Could you check a few things on this model? Use its own coordinates, in mm. A direction names the side the tool comes from. Give positions to 0.01 mm unless a question says otherwise; leave off trailing zeros. Write each loop counter-clockwise with the first axis right and the second up, starting at its lowest first coordinate (ties: lowest second). Pieces come first, ordered by that corner, then holes. Notation, with made-up numbers: (-17.5, 53.5) - (2.5, 53.5) arc R14 cw to (2.5, 78.5) - close; hole circle Ø5 at (86.25, -39). An arc over 180 degrees is marked (long way). Use one line per item in the form item = value.
```python
from build123d import *

# Parameters (mm, degrees)
SKETCH1_W           = 17.145
SKETCH1_H           = 17.145
BOSS_EXTRUDE1_DEPTH = 5.08
SKETCH2_R           = 1.27
CUT_EXTRUDE1_DEPTH  = 25.773139688
SKETCH3_R           = 2.54
CUT_EXTRUDE4_DEPTH  = 2.54
SKETCH4_W           = 6.307704678
SKETCH4_H           = 17.145
BOSS_EXTRUDE2_DEPTH = 17.78
SKETCH5_W           = 2.54
SKETCH5_H           = 17.145
BOSS_EXTRUDE3_DEPTH = 5.08
CHAMFER1_SIZE       = 3.175
BOSS_EXTRUDE4_DEPTH = 2.54
BOSS_EXTRUDE5_DEPTH = 2.54
SKETCH9_W           = 1
SKETCH9_H           = 17.145
CUT_EXTRUDE5_DEPTH  = 17.78
EXTRUDE_1_DEPTH     = 1
EXTRUDE_2_DEPTH     = 1
EXTRUDE_3_DEPTH     = 5.31
CUT_EXTRUDE_1_DEPTH = 44.874772364
CUT_EXTRUDE_2_DEPTH = 44.874772364
EXTRUDE_4_DEPTH     = 2.655
EXTRUDE_5_DEPTH     = 6.915
EXTRUDE_6_DEPTH     = 6.92


with BuildPart() as part:
    # Sketch1 → Boss-Extrude1 (new body)
    with BuildSketch(Plane.XY):
        with Locations((8.5725, -8.5725)):
            Rectangle(SKETCH1_W, SKETCH1_H)
    extrude(amount=BOSS_EXTRUDE1_DEPTH)

    # Sketch2 → Cut-Extrude1 (cut, through all)
    with BuildSketch(Plane(origin=(0, 0, 0), x_dir=(-1, 0, 0), z_dir=(0, 0, -1))):
        with Locations((-8.89, -2.5908)):
            Circle(SKETCH2_R)
        with Locations((-8.89, -14.5288)):
            Circle(SKETCH2_R)
    extrude(amount=-CUT_EXTRUDE1_DEPTH, mode=Mode.SUBTRACT)

    # Sketch3 → Cut-Extrude4 (cut)
    with BuildSketch(Plane(origin=(0, 0, 0), x_dir=(-1, 0, 0), z_dir=(0, 0, -1))):
        with Locations((-8.89, -2.5908)):
            Circle(SKETCH3_R)
        with Locations((-8.89, -14.5288)):
            Circle(SKETCH3_R)
    extrude(amount=-CUT_EXTRUDE4_DEPTH, mode=Mode.SUBTRACT)

    # Sketch4 → Boss-Extrude2 (add)
    with BuildSketch(Plane(origin=(0, 0, 0), x_dir=(-1, 0, 0), z_dir=(0, 0, -1))):
        with Locations((-3.153852339, -8.5725)):
            Rectangle(SKETCH4_W, SKETCH4_H)
    extrude(amount=BOSS_EXTRUDE2_DEPTH)

    # Sketch5 → Boss-Extrude3 (add)
    with BuildSketch(Plane.ZY):
        with Locations((3.81, -8.5725)):
            Rectangle(SKETCH5_W, SKETCH5_H)
    extrude(amount=BOSS_EXTRUDE3_DEPTH)

    # Chamfer1
    chamfer1_edges = [part.edges().sort_by_distance(p)[0] for p in [
        (0, -8.5725, -17.78),
    ]]
    chamfer(chamfer1_edges, length=CHAMFER1_SIZE)

    # Sketch7 → Boss-Extrude4 (add)
    with BuildSketch(Plane(origin=(0, 0, 0), x_dir=(1, 0, 0), z_dir=(0, 1, 0))):
        Polygon((-5.08, -2.54), (0, 14.605), (0, -2.54), align=None)
    extrude(amount=-BOSS_EXTRUDE4_DEPTH)

    # Sketch8 → Boss-Extrude5 (add)
    with BuildSketch(Plane.XZ.offset(17.145)):
        Polygon((0, 2.54), (-5.08, 2.54), (0, -14.605), align=None)
    extrude(amount=-BOSS_EXTRUDE5_DEPTH)

    # Sketch9 → Cut-Extrude5 (cut)
    with BuildSketch(Plane(origin=(0, 0, -17.78), x_dir=(-1, 0, 0), z_dir=(0, 0, -1))):
        with Locations((-5.807704678, -8.5725)):
            Rectangle(SKETCH9_W, SKETCH9_H)
    extrude(amount=-CUT_EXTRUDE5_DEPTH, mode=Mode.SUBTRACT)

    # 草图1 → 凸台-拉伸1 (add)
    with BuildSketch(Plane(origin=(0, 0, 0), x_dir=(1, 0, 0), z_dir=(0, 1, 0))):
        Polygon((17.145, 0), (5.307704678, 0), (5.307704678, 17.78), (3.175, 17.78), (0, 14.605), (-5.08, -2.54), (-5.08, -5.08), (17.145, -5.08), align=None)
    extrude(amount=EXTRUDE_1_DEPTH)

    # 草图2 → 凸台-拉伸2 (add)
    with BuildSketch(Plane.XZ.offset(17.145)):
        Polygon((5.307704678, -17.78), (5.307704678, 0), (17.145, 0), (17.145, 5.08), (-5.08, 5.08), (-5.08, 2.54), (0, -14.605), (3.175, -17.78), align=None)
    extrude(amount=EXTRUDE_2_DEPTH)

    # 草图3 → 凸台-拉伸3 (add)
    with BuildSketch(Plane(origin=(17.145, 0, 0), x_dir=(0, 0, -1), z_dir=(1, 0, 0))):
        Polygon((17.78, -18.145), (35.56, -18.145), (35.56, 1), (17.78, 1), (0, 1), (0, -18.145), align=None)
    extrude(amount=-EXTRUDE_3_DEPTH)

    # 草图4 → 切除-拉伸1 (cut, through all)
    with BuildSketch(Plane(origin=(0, 1, 0), x_dir=(1, 0, 0), z_dir=(0, 1, 0))):
        Polygon((15.015, 35.56), (11.835, 32.38), (11.835, 35.56), align=None)
    extrude(amount=-CUT_EXTRUDE_1_DEPTH, mode=Mode.SUBTRACT)

    # 草图5 → 切除-拉伸2 (cut, through all)
    with BuildSketch(Plane(origin=(0, 1, 0), x_dir=(1, 0, 0), z_dir=(0, 1, 0))):
        Polygon((0, 14.605), (-5.08, -2.54), (5.307704678, -2.54), (5.307704678, 0), (5.307704678, 17.78), (3.175, 17.78), align=None)
    extrude(amount=-CUT_EXTRUDE_2_DEPTH, mode=Mode.SUBTRACT)

    # 草图6 → 凸台-拉伸4 (add, symmetric)
    with BuildSketch(Plane(origin=(0, -8.57, 0), x_dir=(-1, 0, 0), z_dir=(0, -1, 0))):
        Polygon((-11.835, 0), (-11.835, 32.38), (5.08, -2.54), (-5.307704678, -2.54), (-5.307704678, 0), align=None)
    extrude(amount=EXTRUDE_4_DEPTH, both=True)

    # 草图7 → 凸台-拉伸5 (add)
    with BuildSketch(Plane(origin=(0, -5.915, 0), x_dir=(1, 0, 0), z_dir=(0, 1, 0))):
        Polygon((5.307704678, -2.54), (-5.08, -2.54), (5.307704678, 0), align=None)
    extrude(amount=EXTRUDE_5_DEPTH)

    # 草图8 → 凸台-拉伸6 (add)
    with BuildSketch(Plane.XZ.offset(11.225)):
        Polygon((-5.08, 2.54), (5.307704678, 2.54), (5.307704678, 0), align=None)
    extrude(amount=EXTRUDE_6_DEPTH)


solid = part.part
```
1. Imagine slicing it at D-D, the plane y = -15.25. List the corners of the cut face in (x, z) for me (3 decimals), and give its area (3 significant figures).
Response values:
outline = (-5.08, 2.54) - (5.308, 0) - (6.455, 0) - (6.455, 2.54) - (7.845, 2.54) - (7.845, 5.08) - (-5.08, 5.08) - close; (9.935, 2.54) - (11.325, 2.54) - (11.325, 0) - (11.835, 0) - (11.835, -32.38) - (15.015, -35.56) - (17.145, -35.56) - (17.145, 5.08) - (9.935, 5.08) - close
area = 266 mm²
2. If we mould it in two halves opening along Y, with no side actions, what happens to faces 5 (the face through (0.19, -14.64, 1.25)), 6 (the face through (6.467, -1.828, 1.252)), 7 (the face through (13, 1, -11))? For each: pulls with the +Y half, pulls with the -Y half, needs draft (parallel to the pull), parting line crosses it, or undercut.
Response values:
face_5 = needs draft
face_6 = undercut
face_7 = pulls with the +Y half
3. For pin 1 (4.5 mm diameter, centred on x = 8.89, y = -14.53, fed in from -Z); pin 2 (6.5 mm diameter, centred on x = 8.89, y = -2.59, fed in from -Z) (3 decimals); pin 3 (7.5 mm diameter, centred on y = -1, z = -15.5, fed in from -X) (3 decimals), each with a flat end and sliding along its axis, tell me the tip position at first contact or that it passes through.
Response values:
pin_1 = 2.54
pin_2 = -32.685
pin_3 = 11.835
4. Imagine slicing it at C-C, the plane z = -24. List the corners of the cut face in (x, y) for me (3 decimals).
Response values:
outline = (7.776, -11.225) - (11.835, -11.225) - (11.835, -18.145) - (17.145, -18.145) - (17.145, 1) - (11.835, 1) - (11.835, -5.915) - (7.776, -5.915) - close
5. Which directions (+Z, -Z, +X, -X, +Y, -Y) give clear straight access to the entire face, cutting with the end or side of a thin tool? Please do faces 1 (the face through (7, -11.225, -11)), 2 (the face through (8, -1, 2.54)), 3 (the face through (6, -8, 5.08)), 4 (the face through (11.835, -2, -16)).
Response values:
face_1 = -Z, -X, -Y
face_2 = -Z
face_3 = +Z, +X, -X, +Y, -Y
face_4 = -Z, -X, +Y
6. If I drill on line 1 (Y direction, x = 8.89, z = 1.55) (3 decimals); line 2 (Y direction, x = 8.89, z = 3.25) (3 decimals); line 3 (X direction, y = -14.75, z = -12) (3 decimals), over which ranges is the centre line in solid material (lowest first)? Write a range as from..to.
Response values:
line_1 = -18.145..-17.069, -11.989..-5.131, -0.051..1
line_2 = -18.145..-15.799, -13.259..-3.861, -1.321..1
line_3 = 11.835..17.145
7. Imagine slicing it at B-B, the plane y = -6.5. List the corners of the cut face in (x, z) for me (3 decimals), and give its area (3 significant figures).
Response values:
outline = (-5.08, 2.54) - (11.835, -32.38) - (15.015, -35.56) - (17.145, -35.56) - (17.145, 5.08) - (-5.08, 5.08) - close
area = 549 mm²
8. Imagine slicing it at A-A, the plane x = 8.89. List the corners of the cut face in (y, z) for me (3 decimals), and give its area (3 significant figures).
Response values:
outline = (-18.145, 0) - (-17.069, 0) - (-17.069, 2.54) - (-15.799, 2.54) - (-15.799, 5.08) - (-18.145, 5.08) - close; (-13.259, 2.54) - (-11.989, 2.54) - (-11.989, 0) - (-11.225, 0) - (-11.225, -26.3) - (-5.915, -26.3) - (-5.915, 0) - (-5.131, 0) - (-5.131, 2.54) - (-3.861, 2.54) - (-3.861, 5.08) - (-13.259, 5.08) - close; (-1.321, 2.54) - (-0.051, 2.54) - (-0.051, 0) - (1, 0) - (1, 5.08) - (-1.321, 5.08) - close
area = 198 mm²
